Part model, mm, in its own coordinate system. A direction names the side the tool comes from. Coordinates: 2 decimals unless noted, no trailing zeros. Loops run counter-clockwise (first coordinate to the right, second up) from the corner with the lowest first, then second, coordinate; pieces in that order, holes last. Notation, with made-up numbers: (36.25, 32) -> (73.25, 32) arc R23 ccw to (73.25, 59) -> close; hole circle Ø8 at (-12.5, 80.25). An arc over 180 degrees is marked (long way). One line per question, with ' | ' between items. Start each with the question number.
1) 3-axis set-ups, long thin cutter, end or side, ignore diameter. For faces 1 (the face through (54, 5, 54.6)), 2 (the face through (77, 5, -5.4)), 3 (the face through (-1.485, -1.972, 67.535)): which of +Z, -Z, +X, -X, +Y, -Y reach the whole face in a straight line?
2) Probe L1, parallel to X at y = -0.5, z = -17; L2, parallel to X at y = 13.25, z = -28; L3, parallel to Y at x = 1, z = 74. List the from-to ranges inside material, lowest first. Write a range as from..to.
3) Two-plate mould, pull along X, no slides. Class faces 4 (the face through (-76, 5, 8.25)), 5 (the face through (97.552, 12, -19)), 6 (the face through (-67.552, -2, -19)): released by +X, released by -X, zero draft, split by the parting line, or undercut.
4) Cut at B-B (y = 7.25). Count the separate pieces of the cut face and the enclosed holes in it, plus the area to 3 significant figures.
5) Cut at A-A (x = 0). List the corners of the cut face in (y, z).
6) Drop flat-ended pins along their axis: pin 1 (8 mm diameter, centred on x = -58.5, z = 80.5, fed in from -Y); pin 2 (10 mm diameter, centred on x = -36.5, z = 51.5, fed in from +Y); pin 3 (9 mm diameter, centred on x = 19.59, z = 85.84, fed in from +Y); pin 4 (1 mm diameter, centred on y = 12, z = 43, fed in from +X). Give the stop position or say it passes through.
from build123d import *

# Parameters (mm, degrees)
REVOLVE1_ANGLE      = 180
BOSS_EXTRUDE1_DEPTH = 38
BOSS_EXTRUDE2_DEPTH = 38
SKETCH4_R           = 2
SKETCH4_R_2         = 5
CUT_EXTRUDE1_DEPTH  = 5
SKETCH5_W           = 6.35
SKETCH5_H           = 9.5
CUT_EXTRUDE2_DEPTH  = 177.103665874


with BuildPart() as part:
    # Sketch1 → Revolve1 (revolve)
    with BuildSketch(Plane.XY):
        Polygon((-74.551832937, 0), (-74.551832937, 14.28), (-78.551832937, 14.28), (-97.551832937, 14.28), (-97.551832937, 10.28), (-78.551832937, 10.28), (-78.551832937, -4), (-67.551832937, -4), (-67.551832937, 0), align=None)
    revolve(axis=Axis((0, 0, 0), (0, 1, 0)), revolution_arc=REVOLVE1_ANGLE)

    # Sketch3 → Boss-Extrude1 (add)
    with BuildSketch(Plane(origin=(0, 0, 0), x_dir=(-1, 0, 0), z_dir=(0, 0, -1))):
        Polygon((-97.551832937, 14.28), (-74.551832937, 14.28), (-74.551832937, 0), (-67.551832937, 0), (-67.551832937, -4), (-78.551832937, -4), (-78.551832937, 10.28), (-97.551832937, 10.28), align=None)
    extrude(amount=BOSS_EXTRUDE1_DEPTH)

    # Sketch1<2> → Boss-Extrude2 (add)
    with BuildSketch(Plane.XY):
        Polygon((-74.551832937, 0), (-74.551832937, 14.28), (-78.551832937, 14.28), (-97.551832937, 14.28), (-97.551832937, 10.28), (-78.551832937, 10.28), (-78.551832937, -4), (-67.551832937, -4), (-67.551832937, 0), align=None)
    extrude(amount=-BOSS_EXTRUDE2_DEPTH)

    # Sketch4 → Cut-Extrude1 (cut, through all)
    with BuildSketch(Plane(origin=(0, 10.28, 0), x_dir=(-1, 0, 0), z_dir=(0, -1, 0))):
        with Locations((0, -91.551832937)):
            Circle(SKETCH4_R)
        with Locations((-91.551832937, 0)):
            Circle(SKETCH4_R)
        with Locations((91.551832937, 0)):
            Circle(SKETCH4_R)
        with Locations((85.844189649, -19.593376102)):
            Circle(SKETCH4_R_2)
        with Locations((79.331960238, -38.204258511)):
            Circle(SKETCH4_R_2)
        with Locations((68.841695079, -54.899419871)):
            Circle(SKETCH4_R_2)
        with Locations((54.899419871, -68.841695079)):
            Circle(SKETCH4_R_2)
        with Locations((38.204258511, -79.331960238)):
            Circle(SKETCH4_R_2)
        with Locations((19.593376102, -85.844189649)):
            Circle(SKETCH4_R_2)
        with Locations((-19.593376102, -85.844189649)):
            Circle(SKETCH4_R_2)
        with Locations((-38.204258511, -79.331960238)):
            Circle(SKETCH4_R_2)
        with Locations((-54.899419871, -68.841695079)):
            Circle(SKETCH4_R_2)
        with Locations((-68.841695079, -54.899419871)):
            Circle(SKETCH4_R_2)
        with Locations((-79.331960238, -38.204258511)):
            Circle(SKETCH4_R_2)
        with Locations((-85.844189649, -19.593376102)):
            Circle(SKETCH4_R_2)
    extrude(amount=-CUT_EXTRUDE1_DEPTH, mode=Mode.SUBTRACT)

    # Sketch5 → Cut-Extrude2 (cut, through all)
    with BuildSketch(Plane(origin=(78.551832937, 0, 0), x_dir=(0, 0, -1), z_dir=(1, 0, 0))):
        with Locations((28.575, 4.75)):
            Rectangle(SKETCH5_W, SKETCH5_H)
        with Locations((18.575, 4.75)):
            Rectangle(SKETCH5_W, SKETCH5_H)
        with Locations((8.575, 4.75)):
            Rectangle(SKETCH5_W, SKETCH5_H)
        with Locations((-1.425, 4.75)):
            Rectangle(SKETCH5_W, SKETCH5_H)
        with Locations((-11.425, 4.75)):
            Rectangle(SKETCH5_W, SKETCH5_H)
        with Locations((-21.425, 4.75)):
            Rectangle(SKETCH5_W, SKETCH5_H)
        with Locations((-31.425, 4.75)):
            Rectangle(SKETCH5_W, SKETCH5_H)
        with Locations((-41.425, 4.75)):
            Rectangle(SKETCH5_W, SKETCH5_H)
        with Locations((-51.425, 4.75)):
            Rectangle(SKETCH5_W, SKETCH5_H)
        with Locations((-61.425, 4.75)):
            Rectangle(SKETCH5_W, SKETCH5_H)
    extrude(amount=-CUT_EXTRUDE2_DEPTH, mode=Mode.SUBTRACT)


solid = part.part
Reported:
1) face 1: -Z, +X, -X | face 2: +X, -X | face 3: -Z, +Y, -Y
2) L1: x = -78.55..-67.55, 67.55..78.55 | L2: x = -97.55..-74.55, 74.55..97.55 | L3: y = -4..0
3) face 4: zero draft | face 5: released by +X | face 6: undercut
4) separate pieces: 21 | enclosed holes: 0 | area: 688 mm²
5) outline: (-4, 67.55) -> (0, 67.55) -> (0, 74.55) -> (14.28, 74.55) -> (14.28, 89.55) -> (10.28, 89.55) -> (10.28, 78.55) -> (-4, 78.55) -> close; (10.28, 93.55) -> (14.28, 93.55) -> (14.28, 97.55) -> (10.28, 97.55) -> close
6) pin 1: stops at y = 10.28 | pin 2: stops at y = 0 | pin 3: passes through | pin 4: stops at x = 87.81
